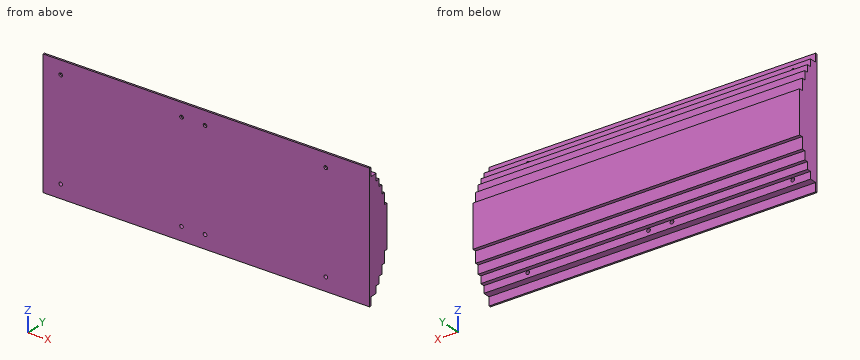
```python
from build123d import *

# Parameters (mm, degrees)
SKETCH1_W                      = 292.1
SKETCH1_H                      = 114.3
EXTRUDE1_DEPTH                 = 1.6002
SKETCH3_W                      = 292.1
SKETCH3_H                      = 99.06
EXTRUDE2_DEPTH                 = 6.35
F_4_CLEARANCE_HOLE1_AT_2_COUNT = 2
F_4_CLEARANCE_HOLE1_AT_2_PITCH = 108.0008
F_4_CLEARANCE_HOLE1_AT_3_COUNT = 2
F_4_CLEARANCE_HOLE1_AT_3_PITCH = 140.584993512
F_4_CLEARANCE_HOLE1_AT_4_COUNT = 2
F_4_CLEARANCE_HOLE1_AT_4_PITCH = 89.99982
F_4_CLEARANCE_HOLE1_AT_5_COUNT = 2
F_4_CLEARANCE_HOLE1_AT_5_PITCH = 253.51541824
F_4_CLEARANCE_HOLE1_AT_6_COUNT = 2
F_4_CLEARANCE_HOLE1_AT_6_PITCH = 157.293864351
F_4_CLEARANCE_HOLE1_AT_7_COUNT = 2
F_4_CLEARANCE_HOLE1_AT_7_PITCH = 129.00152
F_4_CLEARANCE_HOLE1_AT_8_COUNT = 2
F_4_CLEARANCE_HOLE1_AT_8_PITCH = 237.00232
SKETCH4_W                      = 292.1
SKETCH4_H                      = 86.36
EXTRUDE3_DEPTH                 = 3.81
SKETCH5_W                      = 292.1
SKETCH5_H                      = 73.66
EXTRUDE4_DEPTH                 = 3.175
SKETCH6_W                      = 292.1
SKETCH6_H                      = 58.42
EXTRUDE5_DEPTH                 = 3.175
SKETCH7_W                      = 292.1
SKETCH7_H                      = 38.1
EXTRUDE6_DEPTH                 = 3.175
SKETCH8_R                      = 1.63195
CUT_EXTRUDE1_DEPTH             = 177.00338701


with BuildPart() as part:
    # Sketch1 → Extrude1 (new body)
    with BuildSketch(Plane(origin=(0, 0, 0), x_dir=(1, 0, 0), z_dir=(0, 1, 0))):
        with Locations((19.05, 0)):
            Rectangle(SKETCH1_W, SKETCH1_H)
    extrude(amount=EXTRUDE1_DEPTH)

    # Sketch3 → Extrude2 (add)
    with BuildSketch(Plane(origin=(0, 1.6002, 0), x_dir=(-1, 0, 0), z_dir=(0, 1, 0))):
        with Locations((-19.05, 0)):
            Rectangle(SKETCH3_W, SKETCH3_H)
    extrude(amount=EXTRUDE2_DEPTH)

    # Sketch2 → #4 Clearance Hole1 (revolve, cut)
    with BuildSketch(Plane(origin=(125.87732, 1.6002, 44.99864), x_dir=(0, 0, 1), z_dir=(1, 0, 0))):
        Polygon((0, 0), (0, 26.380574487), (1.63195, 25.4), (1.63195, 0), align=None)
    f_4_clearance_hole1 = revolve(axis=Axis((125.87732, 7.9502, 44.99864), (0, -1, 0)), mode=Mode.SUBTRACT)

    # #4 Clearance Hole1 at 2: #4 Clearance Hole1 ×2
    with Locations(*[(-i * F_4_CLEARANCE_HOLE1_AT_2_PITCH, 0, 0) for i in range(1, F_4_CLEARANCE_HOLE1_AT_2_COUNT)]):
        add(f_4_clearance_hole1, mode=Mode.SUBTRACT)

    # #4 Clearance Hole1 at 3: #4 Clearance Hole1 ×2
    with Locations(*[Vector(-0.7682242414518123, 0, -0.6401808454224382) * (i * F_4_CLEARANCE_HOLE1_AT_3_PITCH) for i in range(1, F_4_CLEARANCE_HOLE1_AT_3_COUNT)]):
        add(f_4_clearance_hole1, mode=Mode.SUBTRACT)

    # #4 Clearance Hole1 at 4: #4 Clearance Hole1 ×2
    with Locations(*[(0, 0, -i * F_4_CLEARANCE_HOLE1_AT_4_PITCH) for i in range(1, F_4_CLEARANCE_HOLE1_AT_4_COUNT)]):
        add(f_4_clearance_hole1, mode=Mode.SUBTRACT)

    # #4 Clearance Hole1 at 5: #4 Clearance Hole1 ×2
    with Locations(*[Vector(-0.9348635347125491, 0, -0.35500728367846013) * (i * F_4_CLEARANCE_HOLE1_AT_5_PITCH) for i in range(1, F_4_CLEARANCE_HOLE1_AT_5_COUNT)]):
        add(f_4_clearance_hole1, mode=Mode.SUBTRACT)

    # #4 Clearance Hole1 at 6: #4 Clearance Hole1 ×2
    with Locations(*[Vector(-0.8201306550169548, 0, -0.5721762916282541) * (i * F_4_CLEARANCE_HOLE1_AT_6_PITCH) for i in range(1, F_4_CLEARANCE_HOLE1_AT_6_COUNT)]):
        add(f_4_clearance_hole1, mode=Mode.SUBTRACT)

    # #4 Clearance Hole1 at 7: #4 Clearance Hole1 ×2
    with Locations(*[(-i * F_4_CLEARANCE_HOLE1_AT_7_PITCH, 0, 0) for i in range(1, F_4_CLEARANCE_HOLE1_AT_7_COUNT)]):
        add(f_4_clearance_hole1, mode=Mode.SUBTRACT)

    # #4 Clearance Hole1 at 8: #4 Clearance Hole1 ×2
    with Locations(*[(-i * F_4_CLEARANCE_HOLE1_AT_8_PITCH, 0, 0) for i in range(1, F_4_CLEARANCE_HOLE1_AT_8_COUNT)]):
        add(f_4_clearance_hole1, mode=Mode.SUBTRACT)

    # Sketch4 → Extrude3 (add)
    with BuildSketch(Plane(origin=(0, 7.9502, 0), x_dir=(-1, 0, 0), z_dir=(0, 1, 0))):
        with Locations((-19.05, 0)):
            Rectangle(SKETCH4_W, SKETCH4_H)
    extrude(amount=EXTRUDE3_DEPTH)

    # Sketch5 → Extrude4 (add)
    with BuildSketch(Plane(origin=(0, 11.7602, 0), x_dir=(-1, 0, 0), z_dir=(0, 1, 0))):
        with Locations((-19.05, 0)):
            Rectangle(SKETCH5_W, SKETCH5_H)
    extrude(amount=EXTRUDE4_DEPTH)

    # Sketch6 → Extrude5 (add)
    with BuildSketch(Plane(origin=(0, 14.9352, 0), x_dir=(-1, 0, 0), z_dir=(0, 1, 0))):
        with Locations((-19.05, 0)):
            Rectangle(SKETCH6_W, SKETCH6_H)
    extrude(amount=EXTRUDE5_DEPTH)

    # Sketch7 → Extrude6 (add)
    with BuildSketch(Plane(origin=(0, 18.1102, 0), x_dir=(-1, 0, 0), z_dir=(0, 1, 0))):
        with Locations((-19.05, 0)):
            Rectangle(SKETCH7_W, SKETCH7_H)
    extrude(amount=EXTRUDE6_DEPTH)

    # Sketch8 → Cut-Extrude1 (cut, through all)
    with BuildSketch(Plane.XZ):
        with Locations(Location((125.87732, -45.00118, 0), (0, 0, 90))):
            Circle(SKETCH8_R)
        with Locations(Location((17.87652, -45.00118, 0), (0, 0, 90))):
            Circle(SKETCH8_R)
        with Locations(Location((-3.1242, -45.00118, 0), (0, 0, 90))):
            Circle(SKETCH8_R)
        with Locations(Location((-111.125, -45.00118, 0), (0, 0, 90))):
            Circle(SKETCH8_R)
        with Locations(Location((-111.125, 45.00118, 0), (0, 0, 270))):
            Circle(SKETCH8_R)
        with Locations(Location((-3.1242, 45.00118, 0), (0, 0, 270))):
            Circle(SKETCH8_R)
        with Locations(Location((17.87652, 45.00118, 0), (0, 0, 270))):
            Circle(SKETCH8_R)
        with Locations(Location((125.87732, 45.00118, 0), (0, 0, 270))):
            Circle(SKETCH8_R)
    extrude(amount=-CUT_EXTRUDE1_DEPTH, mode=Mode.SUBTRACT)


solid = part.part
```
Can you work these out from the model? Positions are in its coordinate system, mm. Give positions to 0.01 mm unless a question says otherwise; leave off trailing zeros. Loops run counter-clockwise (first coordinate to the right, second up) from the corner with the lowest first, then second, coordinate; pieces in that order, holes last. Notation, with made-up numbers: M 82.25,22.25 L 92.25,22.25 A9 ccw 92.25,36.25 Z; hole C 50.25,18.5 d4. An arc over 180 degrees is marked long. One line per question, with ' | ' between items. Start each with the question number.
Q1. If we section it at A-A (x = 84): Please give me the cut outline in (y, z).
Q2. For pin 1 Ø2.5 at (x, y) = (67.5, 19) entering from -Z; pin 2 Ø5 at (x, z) = (86, 25.5) entering from +Y; pin 3 Ø1 at (x, y) = (-33, 16.5) entering from +Z, each with a flat end and sliding along its axis, tell me the tip position at first contact or that it passes through.
Q3. If I drill on line 1 (Z direction, x = 0, y = 5.25); line 2 (Z direction, x = -46, y = 9.75); line 3 (Y direction, x = 41, z = 47), over which ranges is the centre line in solid material (lowest first)? Write a range as from..to.
Q4. If we section it at B-B (z = -32): Please give me the cut outline in (x, y), plus the area to 3 significant figures.
Computed:
1) outline: M 0,-57.15 L 1.6,-57.15 L 1.6,-49.53 L 7.95,-49.53 L 7.95,-43.18 L 11.76,-43.18 L 11.76,-36.83 L 14.94,-36.83 L 14.94,-29.21 L 18.11,-29.21 L 18.11,-19.05 L 21.29,-19.05 L 21.29,19.05 L 18.11,19.05 L 18.11,29.21 L 14.94,29.21 L 14.94,36.83 L 11.76,36.83 L 11.76,43.18 L 7.95,43.18 L 7.95,49.53 L 1.6,49.53 L 1.6,57.15 L 0,57.15 Z
2) pin 1: stops at z = -29.21 | pin 2: stops at y = 18.11 | pin 3: stops at z = 29.21
3) line 1: z = -49.53..49.53 | line 2: z = -43.18..43.18 | line 3: y = 0..7.95
4) outline: M -127,0 L 165.1,0 L 165.1,14.94 L -127,14.94 Z | area: 4,360 mm²
